Build history of the part. All positions in model axes, mm. Face numbers are marked on the shaded views. A direction names the side the tool comes from. Round coordinates to 2 decimals unless told otherwise and drop trailing zeros. Use a Markdown table: item, result. Add a question column.
Item 1: Probe L1, parallel to Z at x = 0, y = 1.65; L2, parallel to Z at x = -32, y = 19.5; L3, parallel to X at y = 9.5, z = -60. List the from-to ranges inside material, lowest first.
Item 2: Two-plate mould, pull along X, no slides. Class the marked faces 1, 2 and 3: released by +X, released by -X, zero draft, split by the parting line, or undercut.
Item 3: Pin check, flat tips, straight feed: pin 1 (4 mm diameter, centred on y = 10, z = 30.5, fed in from -X); pin 2 (10 mm diameter, centred on x = -37.5, y = 24, fed in from +Z); pin 3 (8 mm diameter, centred on y = 15.5, z = 51, fed in from +X). Stop position of each tip, or through.
Item 4: 3-axis set-ups, long thin cutter, end or side, ignore diameter. For the marked faces 4 and 5: which of +Z, -Z, +X, -X, +Y, -Y reach the whole face in a straight line?
Item 5: Slice it at A-A, the plane y = 8. State how many separate pieces and enclosed holes the cut face has, plus the area to 3 significant figures.
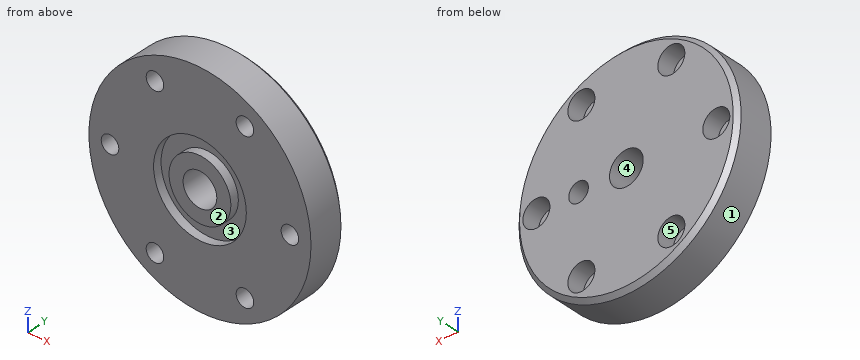
from build123d import *

# Parameters (mm, degrees)
SKETCH1_R                               = 79
SKETCH1_R_2                             = 12
BOSS_EXTRUDE1_DEPTH                     = 27
CBORE_FOR_M5_HEX_HEAD_BOLT1_D           = 12.5
CBORE_FOR_M5_HEX_HEAD_BOLT1_CBORE_D     = 19.25
CBORE_FOR_M5_HEX_HEAD_BOLT1_CBORE_DEPTH = 12.5
F_1_0MM_DOWEL_HOLE1_D                   = 14
F_1_0MM_DOWEL_HOLE1_DEPTH               = 17
F_1_0MM_DOWEL_HOLE1_TIP                 = 4.206024333
SKETCH8_R                               = 33
SKETCH8_R_2                             = 22
CUT_EXTRUDE1_DEPTH                      = 6
CHAMFER1_SIZE                           = 3


with BuildPart() as part:
    # Sketch1 → Boss-Extrude1 (new body)
    with BuildSketch(Plane(origin=(0, 0, 0), x_dir=(1, 0, 0), z_dir=(0, 1, 0))):
        Circle(SKETCH1_R)
        Circle(SKETCH1_R_2, mode=Mode.SUBTRACT)
    extrude(amount=BOSS_EXTRUDE1_DEPTH)

    # CBORE for M5 Hex Head Bolt1 (through all)
    with Locations(Plane(origin=(0, 27, 0), x_dir=(1, 0, 0), z_dir=(0, 1, 0))):
        with Locations((32, 55.425625842), (64, 0), (32, -55.425625842), (-32, -55.425625842), (-64, 0), (-32, 55.425625842), (0, 0)):
            CounterBoreHole(CBORE_FOR_M5_HEX_HEAD_BOLT1_D / 2, CBORE_FOR_M5_HEX_HEAD_BOLT1_CBORE_D / 2, CBORE_FOR_M5_HEX_HEAD_BOLT1_CBORE_DEPTH)

    # Ø1.0mm Dowel Hole1
    with Locations(Plane(origin=(0, 27, 0), x_dir=(1, 0, 0), z_dir=(0, 1, 0))):
        with Locations((34, 0)):
            Hole(F_1_0MM_DOWEL_HOLE1_D / 2, depth=F_1_0MM_DOWEL_HOLE1_DEPTH)
            with Locations((0, 0, -(F_1_0MM_DOWEL_HOLE1_DEPTH + F_1_0MM_DOWEL_HOLE1_TIP / 2))):  # 118° drill point
                Cone(0, F_1_0MM_DOWEL_HOLE1_D / 2, F_1_0MM_DOWEL_HOLE1_TIP, mode=Mode.SUBTRACT)

    # Sketch8 → Cut-Extrude1 (cut)
    with BuildSketch(Plane(origin=(0, 0, 0), x_dir=(1, 0, 0), z_dir=(0, 1, 0))):
        Circle(SKETCH8_R)
        Circle(SKETCH8_R_2, mode=Mode.SUBTRACT)
    extrude(amount=CUT_EXTRUDE1_DEPTH, mode=Mode.SUBTRACT)

    # Chamfer1
    chamfer1_edges = [part.edges().sort_by_distance(p)[0] for p in [
        (-79, 27, 0),
    ]]
    chamfer(chamfer1_edges, length=CHAMFER1_SIZE)


solid = part.part
Check sheet entries:
| question | item | result |
|---|---|---|
| 1 | L1 | -79 to -33, -22 to -12, 12 to 22, 33 to 79 |
| 1 | L2 | -72.23 to -65.05, -45.8 to 45.8, 65.05 to 72.23 |
| 1 | L3 | -51.39 to -36.26, -27.74 to 27.74, 36.26 to 51.39 |
| 2 | face 1 | split by the parting line |
| 2 | face 2 | zero draft |
| 2 | face 3 | undercut |
| 3 | pin 1 | x = -73.68 |
| 3 | pin 2 | z = 72.01 |
| 3 | pin 3 | x = 63.5 |
| 4 | face 4 | +Y, -Y |
| 4 | face 5 | +Y |
| 5 | separate pieces | 1 |
| 5 | enclosed holes | 8 |
| 5 | area | 18,400 mm2 |
